For this review, take the finished solid that the model builds, in its own axes (mm). A direction names the side the tool comes from. Give positions to 0.01 mm unless a question says otherwise; leave off trailing zeros. Order: outer loops, then holes, each group sorted by start corner. A loop starts at its lowest first (then second) coordinate and runs counter-clockwise, first axis right, second up. Notation, with made-up numbers: (-16.75, 16) - (28.25, 16) arc R20 cw to (28.25, 38) - close; hole circle Ø9 at (-30, 31). An arc over 180 degrees is marked (long way). Use a Markdown table: item, result. Add a question column.
1) We need section C-C on x = 5. Write out the cut boundary in (y, z) (3 decimals), then the cut area to 3 significant figures.
2) Wall thickness on L1, parallel to Y at x = 0.75, z = 0 (3 decimals); L2, parallel to Y at x = 12, z = 2; L3, parallel to X at y = 14.5, z = -6.5: over which ranges is each line inside the solid? List them lowest first.
3) Mouldability with a two-part tool opening along Z and no side actions: class faces 5 (the face through (15, 16.4, -2.9)), 6 (the face through (7.75, -4.88, 15.5)), 7 (the face through (3.5, 3.4, 3.9)) as released by +Z, released by -Z, zero draft, split by the parting line, or undercut.
4) Machinability: for faces 1 (the face through (7.306, -4.864, 15.446)), 2 (the face through (13.27, -6.32, -15.24)), 3 (the face through (0, 16.4, -2.9)), 4 (the face through (1.774, -4.956, -15.738)), which of the approach directions +Z, -Z, +X, -X, +Y, -Y give a long, thin tool a straight path to every point of the face, cutting with its end or side? Answer none if there is none.
5) Clearance check with flat-ended pins moving along their axes: P1, Ø4, axis at y = -7, z = 1.5, coming from the -X side; P2, Ø5, axis at y = 11.5, z = -9, coming from the +X side; P3, Ø6, axis at x = 8.5, z = 15.5, coming from the +Y side; P4, Ø1, axis at x = 5, y = 7.5, coming from the -Z side. State where each tip first meets the part, or that it passes through.
```python
from build123d import *

# Parameters (mm, degrees)
SKETCH2_R           = 20
BOSS_EXTRUDE1_DEPTH = 15
SKETCH3_R           = 16.5
SKETCH3_R_2         = 5
CUT_EXTRUDE1_DEPTH  = 3.5
CUT_EXTRUDE2_START  = -3.5
SKETCH4_R           = 16.5
SKETCH4_R_2         = 5
CUT_EXTRUDE2_DEPTH  = 3.5
SKETCH6_R           = 3.125
CUT_EXTRUDE3_DEPTH  = 33.015621187


with BuildPart() as part:
    # Sketch2 → Boss-Extrude1 (new body)
    with BuildSketch(Plane(origin=(0, 0, 0), x_dir=(0, 0, -1), z_dir=(1, 0, 0))):
        Circle(SKETCH2_R)
    extrude(amount=BOSS_EXTRUDE1_DEPTH)

    # Sketch3 → Cut-Extrude1 (cut)
    with BuildSketch(Plane(origin=(15, 0, 0), x_dir=(0, 0, -1), z_dir=(1, 0, 0))):
        Circle(SKETCH3_R)
        Circle(SKETCH3_R_2, mode=Mode.SUBTRACT)
    extrude(amount=-CUT_EXTRUDE1_DEPTH, mode=Mode.SUBTRACT)

    # Sketch4 → Cut-Extrude2 (cut)
    with BuildSketch(Plane.ZY.offset(CUT_EXTRUDE2_START)):
        with Locations(Location((0, 0, 0), (0, 0, 180))):
            Circle(SKETCH4_R)
        with Locations(Location((0, 0, 0), (0, 0, 180))):
            Circle(SKETCH4_R_2, mode=Mode.SUBTRACT)
    extrude(amount=CUT_EXTRUDE2_DEPTH, mode=Mode.SUBTRACT)

    # Sketch6 → Cut-Extrude3 (cut, through all)
    with BuildSketch(Plane(origin=(15, 0, 0), x_dir=(0, 0, -1), z_dir=(1, 0, 0))):
        Circle(SKETCH6_R)
    extrude(amount=-CUT_EXTRUDE3_DEPTH, mode=Mode.SUBTRACT)

    # Sketch7 → Cut-Revolve3 (revolve, cut)
    with BuildSketch(Plane(origin=(0, 0, 0), x_dir=(1, 0, 0), z_dir=(0, 1, 0)), mode=Mode.PRIVATE) as cut_revolve3_sk:
        Polygon((3.5, 20), (7.5, 16), (11.5, 20), align=None)
    revolve(cut_revolve3_sk.sketch.rotate(Axis((0, 0, 0), (1, 0, 0)), 180), axis=Axis((0, 0, 0), (1, 0, 0)), mode=Mode.SUBTRACT)


solid = part.part
```
Checked values:
| question | item | result |
|---|---|---|
| 1 | outline | circle Ø37 at (0, 0); hole circle Ø6.25 at (0, 0) |
| 1 | area | 1,040 mm² |
| 2 | L1 | -20 to -16.5, -5 to -3.125, 3.125 to 5, 16.5 to 20 |
| 2 | L2 | -19.9 to -16.38, -4.58 to -2.4, 2.4 to 4.58, 16.38 to 19.9 |
| 2 | L3 | 3.5 to 11.5 |
| 3 | face 5 | zero draft |
| 3 | face 6 | split by the parting line |
| 3 | face 7 | undercut |
| 4 | face 1 | none |
| 4 | face 2 | +X |
| 4 | face 3 | +Z, -Z, -X, +Y, -Y |
| 4 | face 4 | -X |
| 5 | P1 | x = 3.5 |
| 5 | P2 | x = 15 |
| 5 | P3 | y = 13.74 |
| 5 | P4 | z = -17.5 |
